Can you work these out from the model? Positions are in its coordinate system, mm. Face numbers are marked on the shaded views. A direction names the side the tool comes from. Give positions to 0.01 mm unless a question says otherwise; leave off trailing zeros. Loops run counter-clockwise (first coordinate to the right, second up) from the corner with the lowest first, then second, coordinate; pieces in that order, holes last. Notation, with made-up numbers: M -17.5,49.25 L 39.5,49.25 A19 cw 39.5,75.25 Z; hole C 56.5,-4 d4. An arc over 180 degrees is marked long. Answer as a JSON object with one key per item and string values.
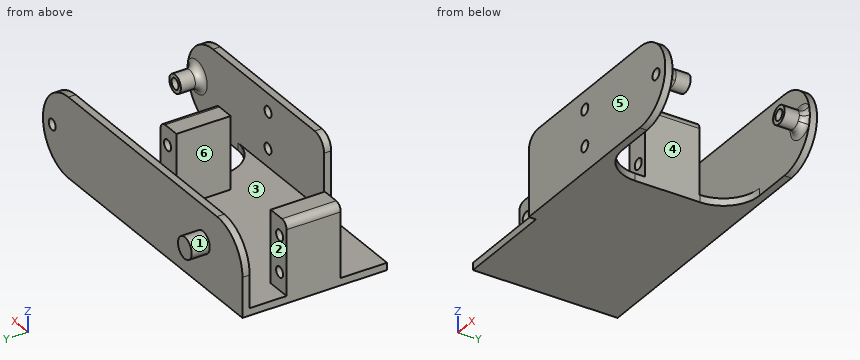
```python
from build123d import *

# Parameters (mm, degrees)
SKETCH_W        = 54.3
SKETCH_H        = 38
PAD_DEPTH       = 2
SKETCH003_W     = 6.85
SKETCH003_H     = 15
PAD001_DEPTH    = 20
SKETCH010_W     = 6.85
SKETCH010_H     = 15
PAD002_DEPTH    = 20
SKETCH004_R     = 1.5
POCKET_DEPTH    = 15
SKETCH002_R     = 1.5
POCKET001_DEPTH = 15
SKETCH005_R     = 1.5
PAD003_DEPTH    = 2
SKETCH007_R     = 1.5
PAD004_DEPTH    = 2
SKETCH006_R     = 2.95
PAD005_DEPTH    = 5
SKETCH008_R     = 2.5
SKETCH008_R_2   = 1.5
PAD006_DEPTH    = 6
SKETCH009_R     = 2.5
SKETCH009_R_2   = 1.5
PAD007_DEPTH    = 6
FILLET_R        = 10
FILLET001_R     = 10
FILLET002_R     = 2
FILLET003_R     = 2
FILLET004_R     = 2
FILLET005_R     = 2
FILLET006_R     = 4


with BuildPart() as part:
    # Sketch → Pad (new body)
    with BuildSketch(Plane.XY.offset(2)):
        Rectangle(SKETCH_W, SKETCH_H)
    extrude(amount=PAD_DEPTH)

    # Sketch003 (on Face6 of Pad) → Pad001 (join)
    with BuildSketch(Plane.XY.offset(4)):
        with Locations((23.725, 1.3)):
            Rectangle(SKETCH003_W, SKETCH003_H)
    extrude(amount=PAD001_DEPTH)

    # Sketch010 (on Face5 of Pad001) → Pad002 (join)
    with BuildSketch(Plane.XY.offset(4)):
        with Locations((-23.725, 1.3)):
            Rectangle(SKETCH010_W, SKETCH010_H)
    extrude(amount=PAD002_DEPTH)

    # Sketch004 (on Face12 of Pad002) → Pocket (cut)
    with BuildSketch(Plane(origin=(0, -6.2, 2), x_dir=(1, 0, 0), z_dir=(0, -1, 0))):
        with Locations((-24.15, 7)):
            Circle(SKETCH004_R)
        with Locations((-24.15, 17)):
            Circle(SKETCH004_R)
    extrude(amount=-POCKET_DEPTH, mode=Mode.SUBTRACT)

    # Sketch002 (on Face11 of Pocket) → Pocket001 (cut)
    with BuildSketch(Plane(origin=(0, -6.2, 2), x_dir=(1, 0, 0), z_dir=(0, -1, 0))):
        with Locations((24.15, 17)):
            Circle(SKETCH002_R)
        with Locations((24.15, 7)):
            Circle(SKETCH002_R)
    extrude(amount=-POCKET001_DEPTH, mode=Mode.SUBTRACT)

    # Sketch005 (on Face1 of Pocket001) → Pad003 (join)
    with BuildSketch(Plane(origin=(0, 19, 2), x_dir=(-1, 0, 0), z_dir=(0, 1, 0))):
        with BuildLine():
            Line((16.15, 22), (-47.85, 22))
            ThreePointArc((-47.85, 22), (-58.85, 11), (-47.85, 0))
            Line((27.15, 0), (-47.85, 0))
            Line((27.15, 0), (27.15, 11))
            ThreePointArc((27.15, 11), (23.928175, 18.778175), (16.15, 22))
        make_face()
        with Locations((-54.85, 11)):
            Circle(SKETCH005_R, mode=Mode.SUBTRACT)
    extrude(amount=PAD003_DEPTH)

    # Sketch007 (on Face2 of Pad003) → Pad004 (join)
    with BuildSketch(Plane(origin=(0, -19, 2), x_dir=(1, 0, 0), z_dir=(0, -1, 0))):
        with BuildLine():
            Line((0, 22), (0, 0))
            Line((0, 0), (47.85, 0))
            ThreePointArc((47.85, 0), (58.85, 11), (47.85, 22))
            Line((0, 22), (47.85, 22))
        make_face()
        with Locations((54.85, 11)):
            Circle(SKETCH007_R, mode=Mode.SUBTRACT)
        with Locations((24.15, 7)):
            Circle(SKETCH007_R, mode=Mode.SUBTRACT)
        with Locations((24.15, 17)):
            Circle(SKETCH007_R, mode=Mode.SUBTRACT)
    extrude(amount=PAD004_DEPTH)

    # Sketch006 (on Face11 of Pad004) → Pad005 (join)
    with BuildSketch(Plane(origin=(0, 21, 2), x_dir=(-1, 0, 0), z_dir=(0, 1, 0))):
        with Locations((10.1, 12)):
            Circle(SKETCH006_R)
    extrude(amount=PAD005_DEPTH)

    # Sketch008 (on Face17 of Pad005) → Pad006 (join)
    with BuildSketch(Plane(origin=(0, -19, 2), x_dir=(-1, 0, 0), z_dir=(0, 1, 0))):
        with Locations((-54.85, 11)):
            Circle(SKETCH008_R)
        with Locations((-54.85, 11)):
            Circle(SKETCH008_R_2, mode=Mode.SUBTRACT)
    extrude(amount=PAD006_DEPTH)

    # Sketch009 (on Face10 of Pad006) → Pad007 (join)
    with BuildSketch(Plane(origin=(0, 19, 2), x_dir=(1, 0, 0), z_dir=(0, -1, 0))):
        with Locations((54.85, 11)):
            Circle(SKETCH009_R)
        with Locations((54.85, 11)):
            Circle(SKETCH009_R_2, mode=Mode.SUBTRACT)
    extrude(amount=PAD007_DEPTH)

    # Fillet
    fillet_edges = [part.edges().sort_by_distance(p)[0] for p in [
        (27.15, -19, 3),
    ]]
    fillet(fillet_edges, radius=FILLET_R)

    # Fillet001
    fillet001_edges = [part.edges().sort_by_distance(p)[0] for p in [
        (27.15, 19, 3),
    ]]
    fillet(fillet001_edges, radius=FILLET001_R)

    # Fillet002
    fillet002_edges = [part.edges().sort_by_distance(p)[0] for p in [
        (52.35, 19, 13),
    ]]
    fillet(fillet002_edges, radius=FILLET002_R)

    # Fillet003
    fillet003_edges = [part.edges().sort_by_distance(p)[0] for p in [
        (57.35, -19, 13),
    ]]
    fillet(fillet003_edges, radius=FILLET003_R)

    # Fillet004
    fillet004_edges = [part.edges().sort_by_distance(p)[0] for p in [
        (27.15, 1.3, 24),
    ]]
    fillet(fillet004_edges, radius=FILLET004_R)

    # Fillet005
    fillet005_edges = [part.edges().sort_by_distance(p)[0] for p in [
        (-27.15, 1.3, 24),
    ]]
    fillet(fillet005_edges, radius=FILLET005_R)

    # Fillet006
    fillet006_edges = [part.edges().sort_by_distance(p)[0] for p in [
        (0, -20, 24),
    ]]
    fillet(fillet006_edges, radius=FILLET006_R)


solid = part.part
```
1) Suppose I cut it at A-A, the plane y = -3.5. Write out the boundary of the cut face in (x, z).
Answer list:
{"outline": "M -27.15,2 L 27.15,2 L 27.15,22 A2 ccw 25.15,24 L 20.3,24 L 20.3,4 L -20.3,4 L -20.3,24 L -25.15,24 A2 ccw -27.15,22 Z; hole C -24.15,9 d3; hole C -24.15,19 d3; hole C 24.15,9 d3; hole C 24.15,19 d3"}
2) Suppose I cut it at D-D, the plane x = 54.85. Write out the boundary of the cut face in (y, z).
Answer list:
{"outline": "M -21,4.51 L -19,4.51 L -19,8.5 A2 cw -17,10.5 L -13,10.5 L -13,11.5 L -21,11.5 Z; M -21,14.5 L -13,14.5 L -13,15.5 L -17,15.5 A2 cw -19,17.5 L -19,21.49 L -21,21.49 Z; M 13,10.5 L 17,10.5 A2 cw 19,8.5 L 19,4.51 L 21,4.51 L 21,11.5 L 13,11.5 Z; M 13,14.5 L 21,14.5 L 21,21.49 L 19,21.49 L 19,17.5 A2 cw 17,15.5 L 13,15.5 Z"}
3) Suppose I cut it at B-B, the plane z = 19. Write out the boundary of the cut face in (x, y).
Answer list:
{"outline": "M -27.15,-6.2 L -25.65,-6.2 L -25.65,8.8 L -27.15,8.8 Z; M -25.37,19 L 57.07,19 L 57.07,21 L -25.37,21 Z; M -22.65,-6.2 L -20.3,-6.2 L -20.3,8.8 L -22.65,8.8 Z; M 0,-21 L 22.65,-21 L 22.65,-19 L 0,-19 Z; M 20.3,-6.2 L 22.65,-6.2 L 22.65,8.8 L 20.3,8.8 Z; M 25.65,-21 L 57.07,-21 L 57.07,-19 L 25.65,-19 Z; M 25.65,-6.2 L 27.15,-6.2 L 27.15,8.8 L 25.65,8.8 Z"}
4) For the marked faces 4, 5 and 6, which set-ups out of +Z, -Z, +X, -X, +Y, -Y let a thin tool reach every point of the face, with its end or its side?
Answer list:
{"face 4": "+Z, -Z, +X", "face 5": "+Z, -Z, +X, -X, -Y", "face 6": "+Z"}
5) If we mould it in two halves opening along X, with no side actions, what happens to the marked faces 1, 2 and 3? For each: +X half, -X half, draft (parallel to the pull), parting line (faces both ways), or undercut.
Answer list:
{"face 1": "parting line", "face 2": "draft", "face 3": "undercut"}
6) Please list where these lines run through material, in increasing order: line 1 along Z through (x, y) = (-24, 5); line 2 along X through (y, z) = (19.7, 13); line 3 along Y through (x, z) = (23, 21). Write a range as from..to.
Answer list:
{"line 1": "2..7.51, 10.49..17.51, 20.49..24", "line 2": "-27.15..53.35, 56.35..58.85", "line 3": "-21..-19, -6.2..8.8, 19..21"}
7) Will these pins go through, and if not, where does the flat tip stop? pin 1 Ø2.5 at (x, z) = (54.85, 13) entering from -Y; pin 2 Ø4 at (x, z) = (11, 11) entering from +Y; pin 3 Ø4 at (x, z) = (-24.15, 19) entering from -Y; pin 4 Ø3 at (x, y) = (20, -7.5) entering from +Z.
Answer list:
{"pin 1": "through", "pin 2": "y = 21", "pin 3": "y = -6.2", "pin 4": "z = 24"}
8) Suppose I cut it at C-C, the plane x = -10.1. Write out the boundary of the cut face in (y, z).
Answer list:
{"outline": "M -19,2 L 21,2 L 21,11.05 L 26,11.05 L 26,16.95 L 21,16.95 L 21,24 L 19,24 L 19,4 L -19,4 Z"}
